from build123d import *

# Parameters (mm, degrees)
SKETCH1_W           = 10
SKETCH1_H           = 38
BOSS_EXTRUDE1_DEPTH = 1.5875
SKETCH2_R           = 3.45
CUT_EXTRUDE1_DEPTH  = 2.5
SKETCH3_R           = 2.875
CUT_EXTRUDE2_DEPTH  = 1.675
SKETCH4_R           = 2.625
CUT_EXTRUDE3_DEPTH  = 4.175


with BuildPart() as part:
    # Sketch1 → Boss-Extrude1 (new body, symmetric)
    with BuildSketch(Plane(origin=(0, 0, 0), x_dir=(1, 0, 0), z_dir=(0, 1, 0))):
        with BuildLine():
            ThreePointArc((-5, 19), (0, 24), (5, 19))
            Line((5, 19), (-5, 19))
        make_face()
        Rectangle(SKETCH1_W, SKETCH1_H)
        with BuildLine():
            Line((5, -19), (-5, -19))
            ThreePointArc((-5, -19), (0, -24), (5, -19))
        make_face()
    extrude(amount=BOSS_EXTRUDE1_DEPTH, both=True)

    # Sketch2 → Cut-Extrude1 (cut)
    with BuildSketch(Plane(origin=(0, 1.5875, 0), x_dir=(1, 0, 0), z_dir=(0, 1, 0))):
        with Locations((0, 19)):
            Circle(SKETCH2_R)
    extrude(amount=-CUT_EXTRUDE1_DEPTH, mode=Mode.SUBTRACT)

    # Sketch3 → Cut-Extrude2 (cut, through all)
    with BuildSketch(Plane(origin=(0, -0.9125, 0), x_dir=(1, 0, 0), z_dir=(0, 1, 0))):
        with Locations((0, 19)):
            Circle(SKETCH3_R)
    extrude(amount=-CUT_EXTRUDE2_DEPTH, mode=Mode.SUBTRACT)

    # Sketch4 → Cut-Extrude3 (cut, through all)
    with BuildSketch(Plane(origin=(0, 1.5875, 0), x_dir=(1, 0, 0), z_dir=(0, 1, 0))):
        with Locations((0, -19)):
            Circle(SKETCH4_R)
    extrude(amount=-CUT_EXTRUDE3_DEPTH, mode=Mode.SUBTRACT)


solid = part.part
Input: part model. Units: mm. Frame: model coordinates. A direction names the side the tool comes from. Round coordinates to 2 decimals unless told otherwise and drop trailing zeros. Order: outer loops, then holes, each group sorted by start corner. A loop starts at its lowest first (then second) coordinate and runs counter-clockwise, first axis right, second up. Notation, with made-up numbers: (15.25, 78.5) - (51.25, 78.5) arc R28 cw to (51.25, 109.5) - close; hole circle Ø5 at (-37.5, 75). An arc over 180 degrees is marked (long way). Answer as a JSON object with one key per item and string values. Group by question number.
(1) Cut plane C-C (y = 0.9). Return loops of the section in (x, z) (3 decimals).
(2) Draft query along X for faces 3 (the face through (-5, 0, 0)), 4 (the face through (0, 0, -24)), 5 (the face through (-0.623, -1.245, -16.193)), 6 (the face through (5, 0, 0)). Return one class per face: released by +X, released by -X, zero draft, split by the parting line, or undercut.
(3) Pin query (flat end, axial travel): P1, Ø1.5, axis at x = 2, y = -1, coming from the +Z side. Return the tip coordinate at first contact, or that it passes through.
(4) Cut plane B-B (z = 20.5). Return loops of the section in (x, y).
(5) Reachability of faces 1 (the face through (-0.45, 0.36, -22.42)), 2 (the face through (0, -1.588, 0)) from +Z, -Z, +X, -X, +Y, -Y: full face, straight path, thin tool, end or side. Return the list, or none.
(6) Cut plane A-A (x = 0). Count the separate pieces of the cut face and the enclosed holes in it, then the cut area to 3 significant figures.
(7) Material intervals for probe 1 along Z at (x, y) = (0, -1.15) (3 decimals); probe 2 along Z at (x, y) = (0, 0.7) (3 decimals); probe 3 along X at (y, z) = (0.9, -19), sorted ascending. Write a range as from..to.
Here are the results:
{
 "1": {"outline": "(-5, -19) arc R5 ccw to (5, -19) - (5, 19) arc R5 ccw to (-5, 19) - close; hole circle Ø6.9 at (0, -19); hole circle Ø5.25 at (0, 19)"},
 "2": {"face 3": "released by -X", "face 4": "split by the parting line", "face 5": "undercut", "face 6": "released by +X"},
 "3": {"P1": "stops at z = 23.84"},
 "4": {"outline": "(-4.77, -1.59) - (-2.15, -1.59) - (-2.15, 1.59) - (-4.77, 1.59) - close; (2.15, -1.59) - (4.77, -1.59) - (4.77, 1.59) - (2.15, 1.59) - close"},
 "5": {"face 1": "+Y", "face 2": "+Z, -Z, +X, -X, -Y"},
 "6": {"separate pieces": "3", "enclosed holes": "0", "area": "115 mm^2"},
 "7": {"probe 1": "z = -24..-21.875, -16.125..16.375, 21.625..24", "probe 2": "z = -24..-22.45, -15.55..16.375, 21.625..24", "probe 3": "x = -5..-3.45, 3.45..5"}
}
